from build123d import *

# Parameters (mm, degrees)
PAD010_DEPTH    = 2.8
FILLET003_R     = 0.4
SKETCH016_R     = 2.5
POCKET008_DEPTH = 2.801
POCKET_DEPTH    = 2.801


with BuildPart() as part:
    # Sketch010 (on Face2 of ShapeBinder009) → Pad010 (new body)
    with BuildSketch(Plane.XZ.offset(25.388718)):
        with BuildLine():
            Line((37.8, 63.127675), (37.8, 60.327675))
            Line((37.8, 60.327675), (23.8, 60.327675))
            ThreePointArc((23.8, 60.327675), (23.4, 59.927675), (23.8, 59.527675))
            Line((23.8, 59.527675), (37.8, 59.527675))
            Line((37.8, 59.527675), (37.8, 44.127675))
            Line((37.8, 44.127675), (23.8, 44.127675))
            ThreePointArc((23.8, 44.127675), (23.4, 43.727675), (23.8, 43.327675))
            Line((23.8, 43.327675), (37.8, 43.327675))
            Line((37.8, 43.327675), (37.8, 40.527675))
            Line((37.8, 40.527675), (35.8, 39.777675))
            Line((35.8, 40.527675), (35.8, 39.777675))
            Line((35.8, 40.527675), (33, 40.527675))
            Line((33, 40.527675), (33, 38.527675))
            Line((33, 38.527675), (25.535898, 40.527675))
            Line((25.535898, 40.527675), (-25.535898, 40.527675))
            Line((-25.535898, 40.527675), (-33, 38.527675))
            Line((-33, 38.527675), (-33, 40.527675))
            Line((-33, 40.527675), (-35.8, 40.527675))
            Line((-35.8, 40.527675), (-35.8, 39.777675))
            Line((-37.8, 40.527675), (-35.8, 39.777675))
            Line((-37.8, 40.527675), (-37.8, 43.327675))
            Line((-37.8, 43.327675), (-23.8, 43.327675))
            ThreePointArc((-23.8, 43.327675), (-23.4, 43.727675), (-23.8, 44.127675))
            Line((-23.8, 44.127675), (-37.8, 44.127675))
            Line((-37.8, 44.127675), (-37.8, 59.527675))
            Line((-37.8, 59.527675), (-23.8, 59.527675))
            ThreePointArc((-23.8, 59.527675), (-23.4, 59.927675), (-23.8, 60.327675))
            Line((-23.8, 60.327675), (-37.8, 60.327675))
            Line((-37.8, 60.327675), (-37.8, 63.127675))
            Line((-35.8, 63.877675), (-37.8, 63.127675))
            Line((-35.8, 63.127675), (-35.8, 63.877675))
            Line((-35.8, 63.127675), (-33, 63.127675))
            Line((-33, 63.127675), (-33, 65.127675))
            Line((-33, 65.127675), (-25.535898, 63.127675))
            Line((-25.535898, 63.127675), (25.535898, 63.127675))
            Line((25.535898, 63.127675), (33, 65.127675))
            Line((33, 65.127675), (33, 63.127675))
            Line((33, 63.127675), (35.8, 63.127675))
            Line((35.8, 63.127675), (35.8, 63.877675))
            Line((35.8, 63.877675), (37.8, 63.127675))
        make_face()
    extrude(amount=-PAD010_DEPTH)

    # Fillet003
    fillet003_edges = [part.edges().sort_by_distance(p)[0] for p in [
        (33, -23.988718, 65.127675),
        (37.8, -23.988718, 63.127675),
        (37.8, -23.988718, 60.327675),
        (37.8, -23.988718, 59.527675),
        (37.8, -23.988718, 44.127675),
        (37.8, -23.988718, 43.327675),
        (37.8, -23.988718, 40.527675),
        (33, -23.988718, 38.527675),
        (-33, -23.988718, 65.127675),
        (-37.8, -23.988718, 63.127675),
        (-37.8, -23.988718, 60.327675),
        (-37.8, -23.988718, 59.527675),
        (-37.8, -23.988718, 44.127675),
        (-37.8, -23.988718, 43.327675),
        (-37.8, -23.988718, 40.527675),
        (-33, -23.988718, 38.527675),
    ]]
    fillet(fillet003_edges, radius=FILLET003_R)

    # Sketch016 (on Face2 of Fillet003) → Pocket008 (cut, through all)
    with BuildSketch(Plane.XZ.offset(25.388718)):
        with Locations((-25, 51.827675)):
            Circle(SKETCH016_R)
        with Locations((25, 51.827675)):
            Circle(SKETCH016_R)
    extrude(amount=-POCKET008_DEPTH, mode=Mode.SUBTRACT)

    # Sketch018 (on Face2 of Pocket008) → Pocket (cut, through all)
    with BuildSketch(Plane.XZ.offset(25.388718)):
        with BuildLine():
            ThreePointArc((-1.75, 60.227675), (-2.75, 59.227675), (-1.75, 58.227675))
            Line((-1.75, 58.227675), (1.75, 58.227675))
            ThreePointArc((1.75, 58.227675), (2.75, 59.227675), (1.75, 60.227675))
            Line((-1.75, 60.227675), (1.75, 60.227675))
        make_face()
        with BuildLine():
            ThreePointArc((-1.75, 45.427675), (-2.75, 44.427675), (-1.75, 43.427675))
            Line((-1.75, 43.427675), (1.75, 43.427675))
            ThreePointArc((1.75, 43.427675), (2.75, 44.427675), (1.75, 45.427675))
            Line((-1.75, 45.427675), (1.75, 45.427675))
        make_face()
    extrude(amount=-POCKET_DEPTH, mode=Mode.SUBTRACT)


solid = part.part
For this review, take the finished solid that the model builds, in its own axes (mm). A direction names the side the tool comes from. Coordinates: 2 decimals unless noted, no trailing zeros. Loops run counter-clockwise (first coordinate to the right, second up) from the corner with the lowest first, then second, coordinate; pieces in that order, holes last. Notation, with made-up numbers: (55, 56.5) - (114, 56.5) arc R16 cw to (114, 74.5) - close; hole circle Ø5 at (5, 46). An arc over 180 degrees is marked (long way). Return JSON: item names as keys, results as strings.
Item 1: Mouldability with a two-part tool opening along Z and no side actions: class faces 1 (the flat face through (37.8, -24, 42)), 2 (the cylindrical face through (-2.75, -24.01, 44.45)), 3 (the flat face through (-36.682, -24.008, 40.109)) as pulls with the +Z half, pulls with the -Z half, needs draft (parallel to the pull), parting line crosses it, or undercut.
Determined:
{"face 1": "needs draft", "face 2": "undercut", "face 3": "pulls with the -Z half"}
Item 2: For line 1 (Z direction, x = 25, y = -23.9); line 2 (X direction, y = -25, z = 53.25); line 3 (X direction, y = -24.8, z = 52), list the stretches that pass through material, from the lowest coordinate up.
Determined:
{"line 1": "z = 40.53 to 43.33, 44.13 to 49.33, 54.33 to 59.53, 60.33 to 63.13", "line 2": "x = -37.8 to -27.06, -22.94 to 22.94, 27.06 to 37.8", "line 3": "x = -37.8 to -27.49, -22.51 to 22.51, 27.49 to 37.8"}
Item 3: Insertion check: pin 1 (1.2 mm diameter, centred on y = -23.5, z = 63.5, fed in from +X); pin 2 (0.8 mm diameter, centred on x = 34, y = -24, fed in from +Z); pin 3 (1.4 mm diameter, centred on x = 34.5, y = -24.5, fed in from -Z). Each pin has a flat end and moves straight along its axis. Give the tip position at first contact, or say it passes through.
Determined:
{"pin 1": "stops at x = 37.8", "pin 2": "stops at z = 63.13", "pin 3": "stops at z = 40.53"}
Item 4: Take a section at A-A (x = -10). Give the boundary of the cut face in (y, z), then the cut area to 3 significant figures.
Determined:
{"outline": "(-25.39, 40.53) - (-22.59, 40.53) - (-22.59, 63.13) - (-25.39, 63.13) - close", "area": "63.3 mm2"}
Item 5: Take a section at B-B (y = -23.6). State how many separate pieces and enclosed holes the cut face has, then the cut area to 3 significant figures.
Determined:
{"separate pieces": "1", "enclosed holes": "4", "area": "1,640 mm2"}
Item 6: For faces 4 (the flat face through (-34, -24, 40.528)), 5 (the flat face through (-31, -24, 43.328)), 6 (the flat face through (31, -24, 44.128)), 7 (the cylindrical face through (2.75, -24.01, 44.41)), 8 (the flat face through (33, -24, 64)), list the 3-axis set-ups (+Z, -Z, +X, -X, +Y, -Y) from which the entire face can be reached by the end or side of a thin tool; tool diameter is ignored.
Determined:
{"face 4": "-Z, +Y, -Y", "face 5": "-X, +Y, -Y", "face 6": "+X, +Y, -Y", "face 7": "+Y, -Y", "face 8": "+Z, +Y, -Y"}
